Source: CAD feature listing. Evaluate the final solid. Frame: model axes, mm. Round coordinates to 2 decimals unless told otherwise and drop trailing zeros. Write each loop counter-clockwise with the first axis right and the second up, starting at its lowest first coordinate (ties: lowest second). Pieces come first, ordered by that corner, then holes. Notation, with made-up numbers: M 79,73 L 135,73 A24 ccw 135,98 Z; hole C 63.5,34 d9. An arc over 180 degrees is marked long. Answer in a Markdown table with one row per item.
Autodesk Inventor part; units mm, degrees
ref_plane "YZ Plane" through (0, 0, 0) normal (1, 0, 0) x (0, 1, 0)
ref_plane "XZ Plane" through (0, 0, 0) normal (0, 1, 0) x (-1, 0, 0)
ref_plane "XY Plane" through (0, 0, 0) normal (0, 0, 1) x (1, 0, 0)
sketch "Sketch1" plane through (0, 0, 0) normal (0, 0, 1) x (1, 0, 0)
  line L0 (0, 0) -> (200, 0)
  line L1 (200, 0) -> (200, 93)
  line L2 (200, 93) -> (0, 93)
  line L3 (0, 93) -> (0, 0)
  dimension "d0" = 93
  dimension "d1" = 200
extrude "Extrusion1" add sketch "Sketch1" along normal blind 6.731
sketch "Sketch2" plane through (0, 0, 6.731) normal (0, 0, 1) x (1, 0, 0)
  line L0 (200, 0) -> (200, 93)
  line L1 (200, 93) -> (0, 93)
  line L2 (0, 93) -> (0, 0)
  line L3 (90, 93) -> (110, 93)
  line L4 (110, 93) -> (110, 86.269)
  line L5 (110, 86.269) -> (90, 86.269)
  line L6 (90, 86.269) -> (90, 93)
  line L7 (0, 66.269) -> (6.731, 66.269)
  line L8 (6.731, 66.269) -> (6.731, 46.269)
  line L9 (6.731, 46.269) -> (0, 46.269)
  line L10 (0, 46.269) -> (0, 66.269)
  line L11 (200, 66.269) -> (193.269, 66.269)
  line L12 (193.269, 66.269) -> (193.269, 46.269)
  line L13 (193.269, 46.269) -> (200, 46.269)
  line L14 (200, 46.269) -> (200, 66.269)
  point P0 (100, 86.269)
  point P1 (100, 93)
  dimension "d5" = 20
  dimension "d6" = 6.731
  dimension "d9" = 20
extrude "Extrusion2" cut sketch "Sketch2" against normal blind 6.731
equation "\"d2\" = THICKB"
equation "\"d6\" = THICKB"
equation "\"d7\" = THICKB"
equation "\"THICKA\" = 3.175"
equation "\"THICKB\" = 6.731"
equation "\"THICKC\" = 12.7"
equation "\"THICKPLY\" = 5"
equation "\"MAGDIA\" = 9.5"
equation "\"BALLDIA\" = 12"
properties part number "Controller_Top"
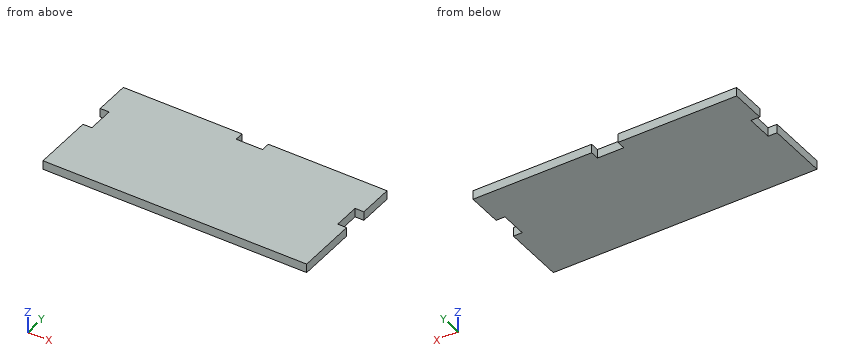
Q1. Material intervals for probe 1 along Y at (x, z) = (90.5, 6.5); probe 2 along X at (y, z) = (62.5, 3), sorted ascending.
Solutions:
| item | result |
|---|---|
| probe 1 | y = 0 to 86.27 |
| probe 2 | x = 6.73 to 193.27 |
Q2. Section A-A (z = 2.5). Return loops of the section in (x, y), and give its area (3 significant figures).
Solutions:
| item | result |
|---|---|
| outline | M 0,0 L 200,0 L 200,46.27 L 193.27,46.27 L 193.27,66.27 L 200,66.27 L 200,93 L 110,93 L 110,86.27 L 90,86.27 L 90,93 L 0,93 L 0,66.27 L 6.73,66.27 L 6.73,46.27 L 0,46.27 Z |
| area | 18,200 mm2 |
Q3. Section B-B (y = 61.5). Return loops of the section in (x, z), and give its area (3 significant figures).
Solutions:
| item | result |
|---|---|
| outline | M 6.73,0 L 193.27,0 L 193.27,6.73 L 6.73,6.73 Z |
| area | 1,260 mm2 |
Q4. Contact query for a flat-ended pin moving along its axis: pin 1 Ø2 at (y, z) = (52.5, 2.5) entering from +X. Output: stop coordinate, or through.
Solutions:
| item | result |
|---|---|
| pin 1 | stops at x = 193.27 |
